The model under review builds one solid part; all positions refer to its coordinate system, in mm. A direction names the side the tool comes from. Coordinates: 2 decimals unless noted, no trailing zeros. Order: outer loops, then holes, each group sorted by start corner. A loop starts at its lowest first (then second) coordinate and runs counter-clockwise, first axis right, second up. Notation, with made-up numbers: (-26.5, -37.5) -> (7.5, -37.5) arc R20 ccw to (7.5, -28.5) -> close; hole circle Ø6 at (-35.75, 87.25). An arc over 180 degrees is marked (long way). Put each result on its own line as item: value.
from build123d import *

# Parameters (mm, degrees)
BOSS_EXTRUDE1_DEPTH                     = 4
CBORE_FOR_M5_HEX_HEAD_BOLT1_D           = 4
CBORE_FOR_M5_HEX_HEAD_BOLT1_CBORE_D     = 8
CBORE_FOR_M5_HEX_HEAD_BOLT1_CBORE_DEPTH = 4.5


with BuildPart() as part:
    # Sketch1 → Boss-Extrude1 (new, symmetric)
    with BuildSketch(Plane.XY):
        Polygon((0, 44.484987277), (0, 0), (48, 0), (48, 50.2), (70, 50.2), (70, 60), (35, 60), (0, 60), align=None)
    extrude(amount=BOSS_EXTRUDE1_DEPTH, both=True)

    # CBORE for M5 Hex Head Bolt1 (through all)
    with Locations(Plane.XY.offset(4)):
        with Locations((6, 10), (6, 54), (51, 55)):
            CounterBoreHole(CBORE_FOR_M5_HEX_HEAD_BOLT1_D / 2, CBORE_FOR_M5_HEX_HEAD_BOLT1_CBORE_D / 2, CBORE_FOR_M5_HEX_HEAD_BOLT1_CBORE_DEPTH)


solid = part.part
Item 1: For faces 1 (the flat face through (59, 50.2, 0)), 2 (the cylindrical face through (5.479, 13.966, 1.781)), 3 (the flat face through (27, 30, 4)), list the 3-axis set-ups (+Z, -Z, +X, -X, +Y, -Y) from which the entire face can be reached by the end or side of a thin tool; tool diameter is ignored.
Answers below:
face 1: +Z, -Z, +X, -Y
face 2: +Z
face 3: +Z, +X, -X, +Y, -Y
Item 2: Consider section B-B on y = 10. Write out the cut boundary in (x, z), and give its area (3 significant figures).
Answers below:
outline: (0, -4) -> (4, -4) -> (4, -0.5) -> (2, -0.5) -> (2, 4) -> (0, 4) -> close; (8, -4) -> (48, -4) -> (48, 4) -> (10, 4) -> (10, -0.5) -> (8, -0.5) -> close
area: 334 mm^2
Item 3: Consider section D-D on z = -1.25. Write out the cut boundary in (x, y), and give its area (3 significant figures).
Answers below:
outline: (0, 0) -> (48, 0) -> (48, 50.2) -> (70, 50.2) -> (70, 60) -> (0, 60) -> close; hole circle Ø4 at (6, 10); hole circle Ø4 at (6, 54); hole circle Ø4 at (51, 55)
area: 3,060 mm^2
Item 4: For line 1 (Y direction, x = 6, z = 2.55); line 2 (Y direction, x = 6, z = -3.25); line 3 (Y direction, x = 51, z = 0.9), list the stretches that pass through material, from the lowest coordinate up. Write a range as from..to.
Answers below:
line 1: 0..6, 14..50, 58..60
line 2: 0..8, 12..52, 56..60
line 3: 50.2..51, 59..60
Item 5: Consider section C-C on z = 2.25. Write out the cut boundary in (x, y), and give its area (3 significant figures).
Answers below:
outline: (0, 0) -> (48, 0) -> (48, 50.2) -> (70, 50.2) -> (70, 60) -> (0, 60) -> close; hole circle Ø8 at (6, 10); hole circle Ø8 at (6, 54); hole circle Ø8 at (51, 55)
area: 2,940 mm^2
Item 6: Consider section A-A on x = 51. Write out the cut boundary in (y, z).
Answers below:
outline: (50.2, -4) -> (53, -4) -> (53, -0.5) -> (51, -0.5) -> (51, 4) -> (50.2, 4) -> close; (57, -4) -> (60, -4) -> (60, 4) -> (59, 4) -> (59, -0.5) -> (57, -0.5) -> close
Item 7: For pin 1 Ø2.5 at (x, y) = (52, 54.5) entering from +Z; pin 2 Ø2.5 at (x, z) = (54.5, -2) entering from -Y; pin 3 Ø4 at (y, z) = (21, 1) entering from +X; pin 4 Ø3 at (x, y) = (51, 55) entering from +Z, all flat-tipped, find the tip position at first contact; note any pin that passes through.
Answers below:
pin 1: z = -0.5
pin 2: y = 50.2
pin 3: x = 48
pin 4: through
Item 8: Mouldability with a two-part tool opening along Y and no side actions: class faces 4 (the cylindrical face through (50.133, 51.095, 1.781)), 5 (the flat face through (24, 0, 0)), 6 (the flat face through (49, 54, -0.5)), 7 (the flat face through (70, 55, 0)) as +Y half, -Y half, draft (parallel to the pull), parting line (faces both ways), or undercut.
Answers below:
face 4: undercut
face 5: -Y half
face 6: undercut
face 7: draft
